from build123d import *

# Parameters (mm, degrees)
SKETCH_W                      = 66.5
SKETCH_H                      = 105
SKETCH_R                      = 2
SKETCH_W_2                    = 21.5
SKETCH_H_2                    = 28.5
PAD_DEPTH                     = 2
SKETCH002_W                   = 18.625
SKETCH002_H                   = 18.625
SKETCH002_W_2                 = 15.625
SKETCH002_H_2                 = 15.625
PAD002_DEPTH                  = 1
SKETCH002_LINEARPATTERN_2_W   = 18.625
SKETCH002_LINEARPATTERN_2_H   = 18.625
SKETCH002_LINEARPATTERN_2_W_2 = 15.625
SKETCH002_LINEARPATTERN_2_H_2 = 15.625
PAD002_LINEARPATTERN_2_DEPTH  = 1
SKETCH002_LINEARPATTERN_3_W   = 18.625
SKETCH002_LINEARPATTERN_3_H   = 18.625
SKETCH002_LINEARPATTERN_3_W_2 = 15.625
SKETCH002_LINEARPATTERN_3_H_2 = 15.625
PAD002_LINEARPATTERN_3_DEPTH  = 1
SKETCH002_LINEARPATTERN_4_W   = 18.625
SKETCH002_LINEARPATTERN_4_H   = 18.625
SKETCH002_LINEARPATTERN_4_W_2 = 15.625
SKETCH002_LINEARPATTERN_4_H_2 = 15.625
PAD002_LINEARPATTERN_4_DEPTH  = 1
LINEARPATTERN002_COUNT        = 9
LINEARPATTERN002_PITCH        = 17.13
SKETCH003_W                   = 150.48745
SKETCH003_H                   = 190.076035
SKETCH003_W_2                 = 66.5
SKETCH003_H_2                 = 105
POCKET_DEPTH                  = 5


with BuildPart() as part:
    # Sketch (on XY_Plane of Origin) → Pad (new body)
    with BuildSketch(Plane.XY):
        Rectangle(SKETCH_W, SKETCH_H)
        with Locations((-21.75, -45)):
            Circle(SKETCH_R, mode=Mode.SUBTRACT)
        with Locations((23.55, 42.7)):
            Circle(SKETCH_R, mode=Mode.SUBTRACT)
        with Locations((-7.5, 0)):
            Rectangle(SKETCH_W_2, SKETCH_H_2, mode=Mode.SUBTRACT)
    extrude(amount=PAD_DEPTH)

    # Sketch002 (on Face12 of Pad) → Pad002 (join)
    with BuildSketch(Plane.XY.offset(2)):
        with Locations((-23.9375, -43.1875)):
            Rectangle(SKETCH002_W, SKETCH002_H)
        with Locations((-23.9375, -43.1875)):
            Rectangle(SKETCH002_W_2, SKETCH002_H_2, mode=Mode.SUBTRACT)
    pad002 = extrude(amount=PAD002_DEPTH)

    # Sketch002 LinearPattern 2 → Pad002 LinearPattern 2 (add)
    with BuildSketch(Plane(origin=(17.125, 0, 2), x_dir=(1, 0, 0), z_dir=(0, 0, 1))):
        with Locations((-23.9375, -43.1875)):
            Rectangle(SKETCH002_LINEARPATTERN_2_W, SKETCH002_LINEARPATTERN_2_H)
        with Locations((-23.9375, -43.1875)):
            Rectangle(SKETCH002_LINEARPATTERN_2_W_2, SKETCH002_LINEARPATTERN_2_H_2, mode=Mode.SUBTRACT)
    pad002_linearpattern_2 = extrude(amount=PAD002_LINEARPATTERN_2_DEPTH)

    # Sketch002 LinearPattern 3 → Pad002 LinearPattern 3 (add)
    with BuildSketch(Plane(origin=(34.25, 0, 2), x_dir=(1, 0, 0), z_dir=(0, 0, 1))):
        with Locations((-23.9375, -43.1875)):
            Rectangle(SKETCH002_LINEARPATTERN_3_W, SKETCH002_LINEARPATTERN_3_H)
        with Locations((-23.9375, -43.1875)):
            Rectangle(SKETCH002_LINEARPATTERN_3_W_2, SKETCH002_LINEARPATTERN_3_H_2, mode=Mode.SUBTRACT)
    pad002_linearpattern_3 = extrude(amount=PAD002_LINEARPATTERN_3_DEPTH)

    # Sketch002 LinearPattern 4 → Pad002 LinearPattern 4 (add)
    with BuildSketch(Plane(origin=(51.375, 0, 2), x_dir=(1, 0, 0), z_dir=(0, 0, 1))):
        with Locations((-23.9375, -43.1875)):
            Rectangle(SKETCH002_LINEARPATTERN_4_W, SKETCH002_LINEARPATTERN_4_H)
        with Locations((-23.9375, -43.1875)):
            Rectangle(SKETCH002_LINEARPATTERN_4_W_2, SKETCH002_LINEARPATTERN_4_H_2, mode=Mode.SUBTRACT)
    pad002_linearpattern_4 = extrude(amount=PAD002_LINEARPATTERN_4_DEPTH)

    # LinearPattern002: Pad002, Pad002 LinearPattern 2, Pad002 LinearPattern 3, Pad002 LinearPattern 4 ×9
    with Locations(*[(0, i * LINEARPATTERN002_PITCH, 0) for i in range(1, LINEARPATTERN002_COUNT)]):
        add(pad002)
        add(pad002_linearpattern_2)
        add(pad002_linearpattern_3)
        add(pad002_linearpattern_4)

    # Sketch003 (on Face131 of MultiTransform) → Pocket (cut)
    with BuildSketch(Plane.XY.offset(3)):
        with Locations((-0.924236, 18.80619)):
            Rectangle(SKETCH003_W, SKETCH003_H)
        Rectangle(SKETCH003_W_2, SKETCH003_H_2, mode=Mode.SUBTRACT)
        Polygon((-16.125, 14.25), (-14.625, 14.25), (1, 14.25), (2.5, 14.25), (3.25, 14.25), (3.25, 0.39), (3.25, -1.115), (3.25, -14.25), (2.5, -14.25), (1, -14.25), (-14.625, -14.25), (-16.125, -14.25), (-18.25, -14.25), (-18.25, -1.115), (-18.25, 0.39), (-18.25, 14.25), align=None)
    extrude(amount=-POCKET_DEPTH, mode=Mode.SUBTRACT)


solid = part.part
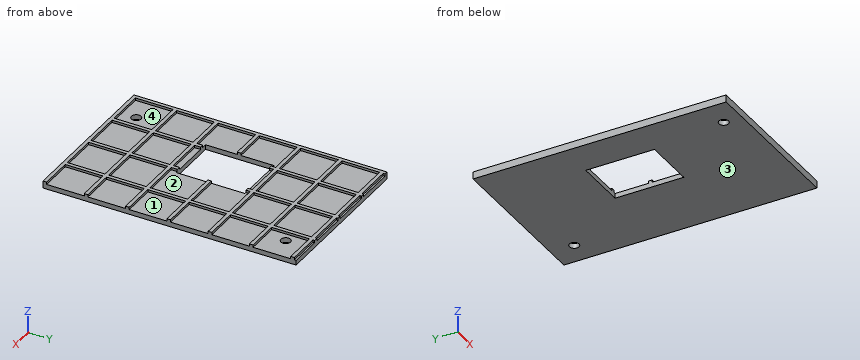
Design review of the part built by this model. Coordinates are the model's own, in mm. Face numbers are marked on the shaded views. A direction names the side the tool comes from. Round coordinates to 2 decimals unless told otherwise and drop trailing zeros. Write each loop counter-clockwise with the first axis right and the second up, starting at its lowest first coordinate (ties: lowest second). Pieces come first, ordered by that corner, then holes. Notation, with made-up numbers: (28.5, 61) - (71.5, 61) arc R26 ccw to (71.5, 100) - close; hole circle Ø11 at (85, 79). An arc over 180 degrees is marked (long way). Return JSON: item names as keys, results as strings. Group by question number.
Item 1: We need section B-B on z = 0.9. Write out the cut boundary in (x, y), and give its area (3 significant figures).
Item 2: We need section A-A on y = -45. Write out the cut boundary in (x, z) (3 decimals), and give its area (3 significant figures).
Item 3: Insertion check: P1, Ø8, axis at x = -8.5, y = 39.5, coming from the +Z side. The pin has a flat end and moves straight along its axis. Give the tip position at first contact, or say it passes through.
Item 4: For probe 1 along X at (y, z) = (42, 2.8) (3 decimals); probe 2 along Y at (x, z) = (-21.75, 1.35); probe 3 along X at (y, z) = (-10.5, 0.35), list the stretches that pass through material, from the lowest coordinate up. Write a range as [from, to].
Item 5: We need section D-D on y = -29. Write out the cut boundary in (x, z) (3 decimals).
Item 6: Machinability: for the marked faces 1 and 2, which of the approach directions +Z, -Z, +X, -X, +Y, -Y give a long, thin tool a straight path to every point of the face, cutting with its end or side? Answer none if there is none.
Item 7: The part is to be moulded in two halves that separate along Y. For the marked faces 3 and 4, say which applies: pulls with the +Y half, pulls with the -Y half, needs draft (parallel to the pull), parting line crosses it, or undercut.
Model answer:
{
 "1": {"outline": "(-33.25, -52.5) - (33.25, -52.5) - (33.25, 52.5) - (-33.25, 52.5) - close; hole circle Ø4 at (-21.75, -45); hole (-18.25, -14.25) - (3.25, -14.25) - (3.25, 14.25) - (-18.25, 14.25) - close; hole circle Ø4 at (23.55, 42.7)", "area": "6,340 mm²"},
 "2": {"outline": "(-33.25, 0) - (-23.75, 0) - (-23.75, 2) - (-31.75, 2) - (-31.75, 3) - (-33.25, 3) - close; (-19.75, 0) - (33.25, 0) - (33.25, 2) - (19.625, 2) - (19.625, 3) - (18.125, 3) - (18.125, 2) - (2.5, 2) - (2.5, 3) - (1, 3) - (1, 2) - (-14.625, 2) - (-14.625, 3) - (-16.125, 3) - (-16.125, 2) - (-19.75, 2) - close", "area": "131 mm²"},
 "3": {"P1": "stops at z = 2"},
 "4": {"probe 1": "x = [-33.25, -31.75], [-16.125, -14.625], [1, 2.5], [18.125, 19.625]", "probe 2": "y = [-52.5, -47], [-43, 52.5]", "probe 3": "x = [-33.25, -18.25], [3.25, 33.25]"},
 "5": {"outline": "(-33.25, 0) - (33.25, 0) - (33.25, 2) - (19.625, 2) - (19.625, 3) - (18.125, 3) - (18.125, 2) - (2.5, 2) - (2.5, 3) - (1, 3) - (1, 2) - (-14.625, 2) - (-14.625, 3) - (-16.125, 3) - (-16.125, 2) - (-31.75, 2) - (-31.75, 3) - (-33.25, 3) - close"},
 "6": {"face 1": "+Z, +X", "face 2": "+Z"},
 "7": {"face 3": "needs draft", "face 4": "undercut"}
}
